```python
from build123d import *

# Parameters (mm, degrees)
ROTOVAT1_ANGLE        = 180
M3_Z_VIT1_D           = 2.5
M3_Z_VIT1_DEPTH       = 19.288970198
M3_Z_VIT1_CSINK_D     = 3.05
M3_Z_VIT1_CSINK_ANGLE = 90


with BuildPart() as part:
    # Skica1 → Rotovat1 (revolve)
    with BuildSketch(Plane.XY):
        Polygon((-358.493859674, -32.75993206), (-357.140613979, -28.995817934), (-359.020013823, -28.311772333), (-360.370342902, -32.067773761), align=None)
    revolve(axis=Axis((-372.880596884, -16.019433279, 0), (-0.342020143, -0.939692621, 0)), revolution_arc=ROTOVAT1_ANGLE)

    # M3 závit1
    with Locations(Plane(origin=(-375.894265461, -24.29837465, 19.236814653), x_dir=(0, 0.999993116, -0.003710613), z_dir=(0.00133078, 0.00371061, 0.99999223))):
        with Locations((0, 0)):
            CounterSinkHole(M3_Z_VIT1_D / 2, M3_Z_VIT1_CSINK_D / 2, depth=M3_Z_VIT1_DEPTH, counter_sink_angle=M3_Z_VIT1_CSINK_ANGLE)


solid = part.part
```
Geometry check sheet. Reference: the model listing, model coordinates, mm. Round coordinates to 2 decimals unless told otherwise and drop trailing zeros. Write item = value, one per line.
Q1. Scan lines: line 1 (Y direction, x = -385, z = 15.25); line 2 (Z direction, x = -385.5, y = -19); line 3 (X direction, y = -20, z = 7). Record each from-to range of solid material in increasing order.
Answer block:
line_1 = -23.11 to -18.86
line_2 = 13.39 to 15.88
line_3 = -393.41 to -391.1
Q2. Release check for a two-part mould opening along Y. For faces 1 (the conical face through (-376.212, -26.303, 17.588)), 2 (the conical face through (-374.879, -22.746, 19.225)), 3 (the cylindrical face through (-376.74, -23.38, 18.06)), 4 (the flat face through (-359, -31, 0)) record: released by +Y, released by -Y, zero draft, split by the parting line, or undercut.
Answer block:
face_1 = released by -Y
face_2 = split by the parting line
face_3 = undercut
face_4 = zero draft
Q3. Depth check by flat-ended pin: pin 1 Ø6 at (y, z) = (-21.5, 11) entering from +X; pin 2 Ø1.5 at (x, y) = (-380.5, -21) entering from +Z; pin 3 Ø4 at (y, z) = (-23, 5.5) entering from -X; pin 4 Ø5 at (y, z) = (-22, 4) entering from -X. Enter the tip coordinate at first touch or a pass-through.
Answer block:
pin_1 = -385.44
pin_2 = 18.65
pin_3 = through
pin_4 = -394.43
